from build123d import *

# Parameters (mm, degrees)
F0_W     = 22
F0_H     = 17
F1_DEPTH = 15
F2_R     = 4.75
F3_DEPTH = 6.5
F4_R     = 3
F5_DEPTH = 21.501
F7_DEPTH = 21.501
F9_D     = 2.5
F9_DEPTH = 5
F9_TIP   = 0.7510757738


with BuildPart() as f1:
    # F0 (on Front) → F1 (new body)
    with BuildSketch(Plane.XZ):
        with Locations((0, 8.5)):
            Rectangle(F0_W, F0_H)
    extrude(amount=-F1_DEPTH)

    # F2 (on face) → F3 (join)
    with BuildSketch(Plane(origin=(0, 15, 0), x_dir=(-1, 0, 0), z_dir=(0, 1, 0))):
        with Locations((0, 7.5)):
            Circle(F2_R)
    extrude(amount=F3_DEPTH)

    # F4 (on face) → F5 (cut, through all)
    with BuildSketch(Plane.XZ):
        with Locations((0, 7.5)):
            Circle(F4_R)
    extrude(amount=-F5_DEPTH, mode=Mode.SUBTRACT)

    # F6 (on face) → F7 (cut, through all)
    with BuildSketch(Plane.XZ):
        Polygon((11, 17), (0, 17), (11, 10.6491470389), align=None)
        Polygon((-11, 10.6491470389), (0, 17), (-11, 17), align=None)
    extrude(amount=-F7_DEPTH, mode=Mode.SUBTRACT)

    # F9
    with Locations(Plane(origin=(7.3612159322, 0, 12.75), x_dir=(0.8660254038, 0, -0.5), z_dir=(0.5, 0, 0.8660254038))):
        with Locations((-6.7057428082, 2.6455062134), (-6.7057428082, 11.6455062134), (2.2942571918, 11.6455062134), (2.2942571918, 2.6455062134)):
            Hole(F9_D / 2, depth=F9_DEPTH)
            with Locations((0, 0, -(F9_DEPTH + F9_TIP / 2))):  # 118° drill point
                Cone(0, F9_D / 2, F9_TIP, mode=Mode.SUBTRACT)


solid = f1.part
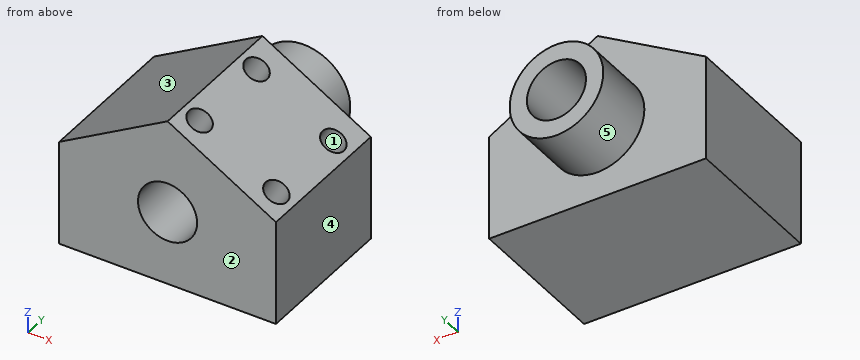
CAD build for the part. Positions are in the model's coordinates, mm. Face numbers are marked on the shaded views. A direction names the side the tool comes from. Give positions to 0.01 mm unless a question says otherwise; leave off trailing zeros. Write each loop counter-clockwise with the first axis right and the second up, starting at its lowest first coordinate (ties: lowest second). Pieces come first, ordered by that corner, then holes. Notation, with made-up numbers: (-0.5, -36.5) - (5.5, -36.5) arc R18 ccw to (5.5, -27.5) - close; hole circle Ø1 at (23, 67). An arc over 180 degrees is marked (long way). Answer as CSV lines item,"result".
Q1. Pull direction Z, two halves, no side cores. Call the marked faces 1, 2 and 3: released by +Z, released by -Z, zero draft, split by the parting line, or undercut.
Result set:
face 1,"undercut"
face 2,"zero draft"
face 3,"released by +Z"
Q2. Band-saw the part on A-A (y = 9.75). Give the cut face in (x, z).
Result set:
outline,"(-11, 0) - (11, 0) - (11, 10.65) - (0, 17) - (-11, 10.65) - close; hole circle Ø6 at (0, 7.5)"
Q3. 3-axis set-ups, long thin cutter, end or side, ignore diameter. For the marked faces 4 and 5: which of +Z, -Z, +X, -X, +Y, -Y reach the whole face in a straight line?
Result set:
face 4,"+Z, -Z, +X, +Y, -Y"
face 5,"+Y"
Q4. Band-saw the part on B-B (z = 9.25). State how many separate pieces and enclosed holes the cut face has, and give its area (3 significant figures).
Result set:
separate pieces,"2"
enclosed holes,"2"
area,"271 mm²"
Q5. Flat gauge pins, fed straight in: pin 1 Ø4 at (y, z) = (18.5, 6) entering from +X; pin 2 Ø3 at (x, y) = (8.5, 14.5) entering from +Z. Where does each tip first touch, or does it go through?
Result set:
pin 1,"x = 4.75"
pin 2,"z = 12.96"
Q6. Drill centre lines: line 1 (Y direction, x = 0, z = 13.5); line 2 (Y direction, x = -5, z = 1.5); line 3 (Z direction, x = -1.5, y = 1.5). Where is each one in solid material? Low to high. Write a range as from..to.
Result set:
line 1,"0..1.4, 3.89..10.4, 12.89..15"
line 2,"0..15"
line 3,"0..4.9, 10.1..16.13"
Q7. Band-saw the part on C-C (z = 3.75). Give the cut face in (x, y).
Result set:
outline,"(-11, 0) - (11, 0) - (11, 15) - (2.92, 15) - (2.92, 21.5) - (-2.92, 21.5) - (-2.92, 15) - (-11, 15) - close"
